```python
from build123d import *

# Parameters (mm, degrees)
F1_DEPTH = 5
F2_SIZE  = 0.5


with BuildPart() as f1:
    # F0 (on Top) → F1 (new body)
    with BuildSketch(Plane.XY):
        with BuildLine():
            Line((28.821813, 3.290897), (-31.235694, 3.290897))
            ThreePointArc((-31.235694, 3.290897), (-40, 0), (-31.235694, -3.290897))
            Line((-31.235694, -3.290897), (28.821813, -3.290897))
            ThreePointArc((28.821813, -3.290897), (42, 0), (28.821813, 3.290897))
        make_face()
        Polygon((-32.15, 1.645448), (-32.15, -1.645448), (-35, -3.290897), (-37.85, -1.645448), (-37.85, 1.645448), (-35, 3.290897), align=None, mode=Mode.SUBTRACT)
        Polygon((39.156922, 0), (37.078461, -3.6), (32.921539, -3.6), (30.843078, 0), (32.921539, 3.6), (37.078461, 3.6), align=None, mode=Mode.SUBTRACT)
    extrude(amount=F1_DEPTH)

    # F2
    f2_edges = [f1.edges().sort_by_distance(p)[0] for p in [
        (-36.425, 2.468172, 5),
        (-33.575, 2.468172, 5),
        (-32.15, 0, 5),
        (-33.575, -2.468172, 5),
        (-36.425, -2.468172, 5),
        (-37.85, 0, 5),
        (42, 0, 5),
        (-1.206941, 3.290897, 5),
        (-40, 0, 5),
        (-1.206941, -3.290897, 5),
        (35, 3.6, 5),
        (38.117691, 1.8, 5),
        (38.117691, -1.8, 5),
        (35, -3.6, 5),
        (31.882309, -1.8, 5),
        (31.882309, 1.8, 5),
        (42, 0, 0),
        (-1.206941, 3.290897, 0),
        (-40, 0, 0),
        (-1.206941, -3.290897, 0),
        (-33.575, 2.468172, 0),
        (-32.15, 0, 0),
        (-33.575, -2.468172, 0),
        (-36.425, -2.468172, 0),
        (-37.85, 0, 0),
        (-36.425, 2.468172, 0),
        (35, 3.6, 0),
        (38.117691, 1.8, 0),
        (38.117691, -1.8, 0),
        (35, -3.6, 0),
        (31.882309, -1.8, 0),
        (31.882309, 1.8, 0),
    ]]
    chamfer(f2_edges, length=F2_SIZE)


solid = f1.part
```
Model file for the job. Use its own axes, mm. A direction names the side the tool comes from. Round coordinates to 2 decimals unless told otherwise and drop trailing zeros. Loops run counter-clockwise (first coordinate to the right, second up) from the corner with the lowest first, then second, coordinate; pieces in that order, holes last. Notation, with made-up numbers: M 78,69 L 135,69 A6 ccw 135,77 Z; hole C 49.5,67 d6. An arc over 180 degrees is marked long. Put each result on its own line as item: value. Start each with the question number.
Item 1: 3-axis set-ups, long thin cutter, end or side, ignore diameter. For faces 1 (the face through (-33.42, -2.67, 0.25)), 2 (the face through (38, -2, 2)), 3 (the face through (-33.42, -2.67, 4.75)): which of +Z, -Z, +X, -X, +Y, -Y reach the whole face in a straight line?
Item 2: Drop flat-ended pins along their axis: P1, Ø3, axis at x = -6.5, z = 3, coming from the -Y side; P2, Ø2, axis at x = 7, z = 3, coming from the +Y side; P3, Ø3, axis at y = 2.5, z = 4, coming from the -X side. Give the stop position or say it passes through.
Item 3: Cut at C-C (x = 14). List the corners of the cut face in (y, z), then the cut area to 3 significant figures.
Item 4: Cut at A-A (x = 35). List the corners of the cut face in (y, z), then the cut area to 3 significant figures.
Item 5: Mould opens along Y. For faces 4 (the face through (-33.472, 2.701, 4.754)), 5 (the face through (-36.528, -2.701, 4.753)), 6 (the face through (4, 0, 0)), 7 (the face through (42, 0, 2)) say: released by +Y, released by -Y, zero draft, split by the parting line, or undercut.
Item 6: Drill centre lines: line 1 along X through (y, z) = (-3, 4.45); line 2 along X through (y, z) = (0.25, 3.15); line 3 along Y through (x, z) = (37.5, 3.85). Where is each one in solid material? Low to high.
Item 7: Cut at B-B (z = 3.6). List the corners of the cut face in (x, y).
Answer block:
1. face 1: -Z
1. face 2: +Z, -Z
1. face 3: +Z
2. P1: y = -3.29
2. P2: y = 3.29
2. P3: x = -39.9
3. outline: M -3.29,0.5 L -2.79,0 L 2.79,0 L 3.29,0.5 L 3.29,4.5 L 2.79,5 L -2.79,5 L -3.29,4.5 Z
3. area: 32.4 mm2
4. outline: M -7,0.5 L -6.5,0 L -4.1,0 L -3.6,0.5 L -3.6,4.5 L -4.1,5 L -6.5,5 L -7,4.5 Z; M 3.6,0.5 L 4.1,0 L 6.5,0 L 7,0.5 L 7,4.5 L 6.5,5 L 4.1,5 L 3.6,4.5 Z
4. area: 33.0 mm2
5. face 4: undercut
5. face 5: undercut
5. face 6: zero draft
5. face 7: split by the parting line
6. line 1: -39 to -35.5, -34.5 to 32.58, 37.42 to 41.32
6. line 2: -39.99 to -37.85, -32.15 to 30.99, 39.01 to 42
6. line 3: -6.54 to -2.87, 2.87 to 6.54
7. outline: M -31.24,-3.29 L 28.82,-3.29 A7 ccw long 28.82,3.29 L -31.24,3.29 A5 ccw long Z; hole M -37.85,-1.65 L -35,-3.29 L -32.15,-1.65 L -32.15,1.65 L -35,3.29 L -37.85,1.65 Z; hole M 30.84,0 L 32.92,-3.6 L 37.08,-3.6 L 39.16,0 L 37.08,3.6 L 32.92,3.6 Z
